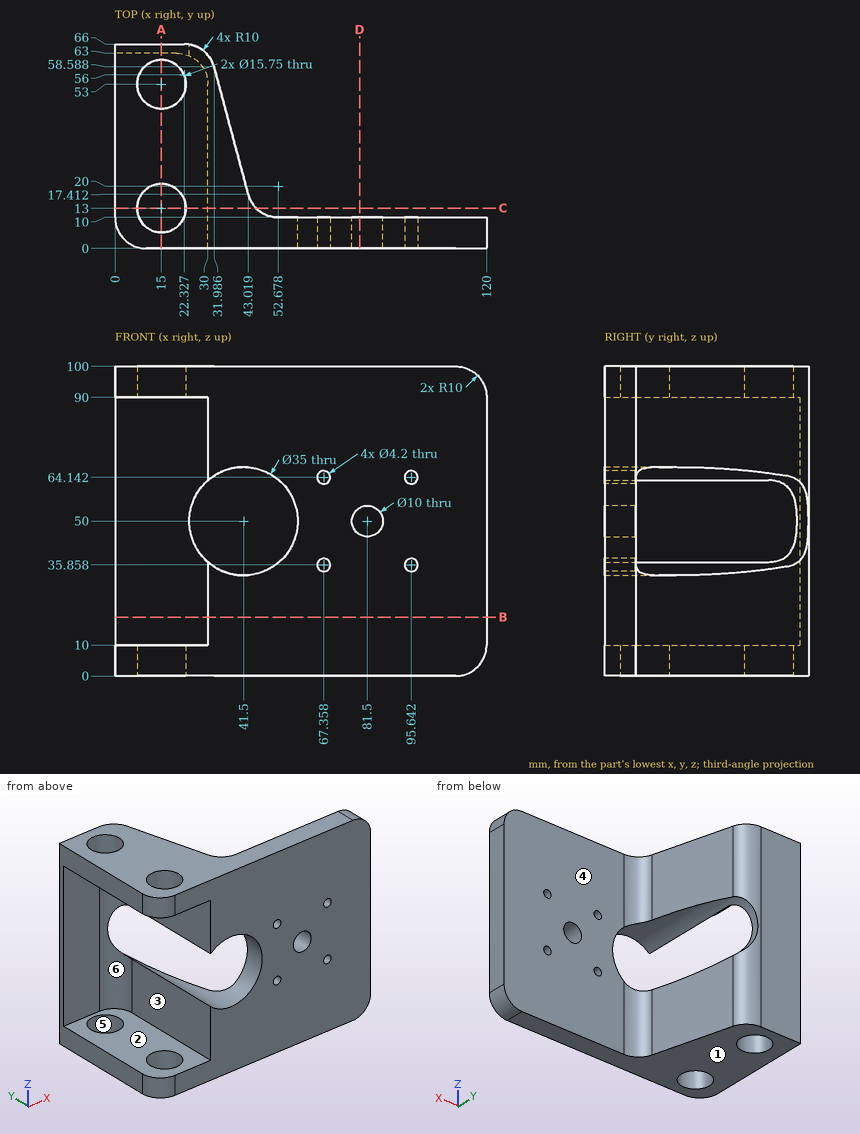
The figure shows three views and two pictorial views of one solid part (mm, origin at its lowest corner). Answer the questions. A direction names the side the tool comes from. Coordinates: 2 decimals unless noted, no trailing zeros. Loops run counter-clockwise (first coordinate to the right, second up) from the corner with the lowest first, then second, coordinate; pieces in that order, holes last.
(1) A tool of negligible diameter and unlimited length cuts with its end or side. For the marked faces 5 and 6, from which of +Z, -Z, +X, -X, +Y, -Y can it reach the whole face along a straight path? Write none if from no direction.
Solution:
face 5: +Z, -Z
face 6: -X, -Y
(2) The part is cut by section B-B (z = 19). Determine the outline of the cut face in (x, y), and give its area (3 significant figures).
Solution:
outline: (0, 63) - (20, 63) arc R10 cw to (30, 53) - (30, 0) - (120, 0) - (120, 10) - (52.68, 10) arc R10 cw to (43.02, 17.41) - (31.99, 58.59) arc R10 ccw to (22.33, 66) - (0, 66) - close
area: 1,430 mm2
(3) Flat-ended cylindrical pins translate along their axes: pin 1 Ø6 at (y, z) = (56.5, 10.5) entering from -X; pin 2 Ø6 at (x, z) = (58, 83) entering from +Y; pin 3 Ø14 at (x, y) = (15, 53) entering from +Z; pin 4 Ø21.5 at (y, z) = (15, 74.5) entering from -X. Find the tip coordinate at first contact, or state that the pin passes through.
Solution:
pin 1: stops at x = 0
pin 2: stops at y = 10
pin 3: passes through
pin 4: stops at x = 30
(4) The part is cut by section D-D (x = 79). Determine the outline of the cut face in (y, z).
Solution:
outline: (0, 0) - (10, 0) - (10, 45.67) - (0, 45.67) - close; (0, 54.33) - (10, 54.33) - (10, 100) - (0, 100) - close
(5) The part is cut by section A-A (x = 15). Determine the outline of the cut face in (y, z) (1 decimal), and give its area (3 significant figures).
Solution:
outline: (0, 0) - (5.1, 0) - (5.1, 10) - (0, 10) - close; (0, 90) - (5.1, 90) - (5.1, 100) - (0, 100) - close; (20.9, 0) - (45.1, 0) - (45.1, 10) - (20.9, 10) - close; (20.9, 90) - (45.1, 90) - (45.1, 100) - (20.9, 100) - close; (60.9, 0) - (66, 0) - (66, 100) - (60.9, 100) - (60.9, 90) - (63, 90) - (63, 10) - (60.9, 10) - close
area: 930 mm2
(6) The part is cut by section C-C (y = 13). Determine the outline of the cut face in (x, z) (1 decimal), and give its area (3 significant figures).
Solution:
outline: (0, 0) - (7.1, 0) - (7.1, 10) - (0, 10) - close; (0, 90) - (7.1, 90) - (7.1, 100) - (0, 100) - close; (22.9, 0) - (45.5, 0) - (45.5, 33) arc R17.5 cw to (30, 36.8) - (30, 10) - (22.9, 10) - close; (22.9, 90) - (30, 90) - (30, 63.2) arc R17.5 cw to (45.5, 67) - (45.5, 100) - (22.9, 100) - close
area: 1,330 mm2
(7) Consider line 1 along Y through (x, z) = (15, 98.25) (1 decimal); line 2 along Z through (x, y) = (27.5, 18.5); line 3 along Z through (x, y) = (35, 6.5). Determine where each line is inside the solid, lowest interval first.
Solution:
line 1: y = 0 to 5.1, 20.9 to 45.1, 60.9 to 66
line 2: z = 0 to 10, 90 to 100
line 3: z = 0 to 33.75, 66.25 to 100
(8) The mould has two halves that part along Z. Classify the marked faces 1, 2, 3 and 4: released by +Z, released by -Z, zero draft, split by the parting line, or undercut.
Solution:
face 1: released by -Z
face 2: undercut
face 3: undercut
face 4: zero draft
